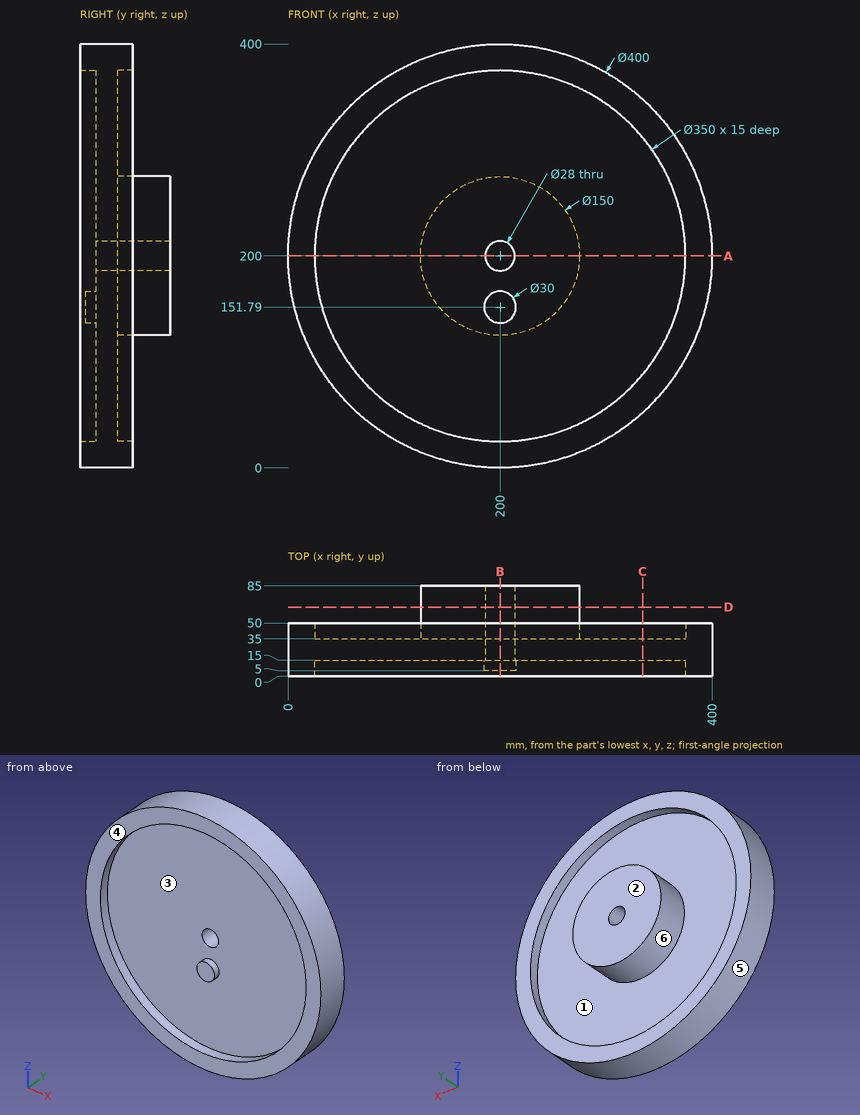
Geometry check sheet. Reference: drawing and pictorial views, mm from the part's lowest x, y, z. A direction names the side the tool comes from. Coordinates: 2 decimals unless noted, no trailing zeros. Order: outer loops, then holes, each group sorted by start corner. A loop starts at its lowest first (then second) coordinate and runs counter-clockwise, first axis right, second up. Notation, with made-up numbers: (55.5, 52) -> (104.5, 52) arc R28 cw to (104.5, 87) -> close; hole circle Ø5 at (74.5, 76). An arc over 180 degrees is marked (long way). Write item = value, one per line. Start each with the question number.
1) Cross-section at A-A (z = 200). Enter the section's corners in (x, y), then the cut area to 3 significant figures.
2) Go/stop test with flat-tipped pins: P1, Ø5, axis at x = 255.5, z = 332, coming from the +Y side; P2, Ø5, axis at y = 74.5, z = 264.5, coming from the -X side; P3, Ø3, axis at x = 210, y = 61.5, coming from the +Z side. Record where each tip stops, or that it passes through.
3) Mould release check, pull along X, two halves, no side actions. Record for the marked faces 4, 5 and 6: +X half, -X half, draft (parallel to the pull), parting line (faces both ways), or undercut.
4) Cross-section at C-C (x = 334.5). Enter the section's corners in (y, z).
5) Material ranges on L1, parallel to Z at x = 200, y = 46; L2, parallel to Z at x = 200, y = 60; L3, parallel to Z at x = 200, y = 30.5, recorded low to high.
6) Access from +Z, -Z, +X, -X, +Y, -Y to the whole of each face (thin tool, end or side, straight path). Record for the marked faces 1, 2 and 3.
7) Cross-section at B-B (x = 200). Enter the section's corners in (y, z), then the cut area to 3 significant figures.
8) Cross-section at D-D (y = 65). Enter the section's corners in (x, z), then the cut area to 3 significant figures.
Ans:
q1.outline = (0, 0) -> (25, 0) -> (25, 15) -> (186, 15) -> (186, 85) -> (125, 85) -> (125, 35) -> (25, 35) -> (25, 50) -> (0, 50) -> close; (214, 15) -> (375, 15) -> (375, 0) -> (400, 0) -> (400, 50) -> (375, 50) -> (375, 35) -> (275, 35) -> (275, 85) -> (214, 85) -> close
q1.area = 15,000 mm²
q2.P1 = 35
q2.P2 = 157.8
q2.P3 = 274.52
q3.face_4 = draft
q3.face_5 = parting line
q3.face_6 = undercut
q4.outline = (0, 51.98) -> (50, 51.98) -> (50, 88.04) -> (35, 88.04) -> (35, 311.96) -> (50, 311.96) -> (50, 348.02) -> (0, 348.02) -> (0, 311.96) -> (15, 311.96) -> (15, 88.04) -> (0, 88.04) -> close
q5.L1 = 0 to 25, 125 to 186, 214 to 275, 375 to 400
q5.L2 = 125 to 186, 214 to 275
q5.L3 = 0 to 186, 214 to 400
q6.face_1 = +Y
q6.face_2 = +Z, -Z, +X, -X, +Y
q6.face_3 = -Y
q7.outline = (0, 0) -> (50, 0) -> (50, 25) -> (35, 25) -> (35, 125) -> (85, 125) -> (85, 186) -> (15, 186) -> (15, 166.79) -> (5, 166.79) -> (5, 136.79) -> (15, 136.79) -> (15, 25) -> (0, 25) -> close; (0, 375) -> (15, 375) -> (15, 214) -> (85, 214) -> (85, 275) -> (35, 275) -> (35, 375) -> (50, 375) -> (50, 400) -> (0, 400) -> close
q7.area = 15,300 mm²
q8.outline = circle Ø150 at (200, 200); hole circle Ø28 at (200, 200)
q8.area = 17,100 mm²
